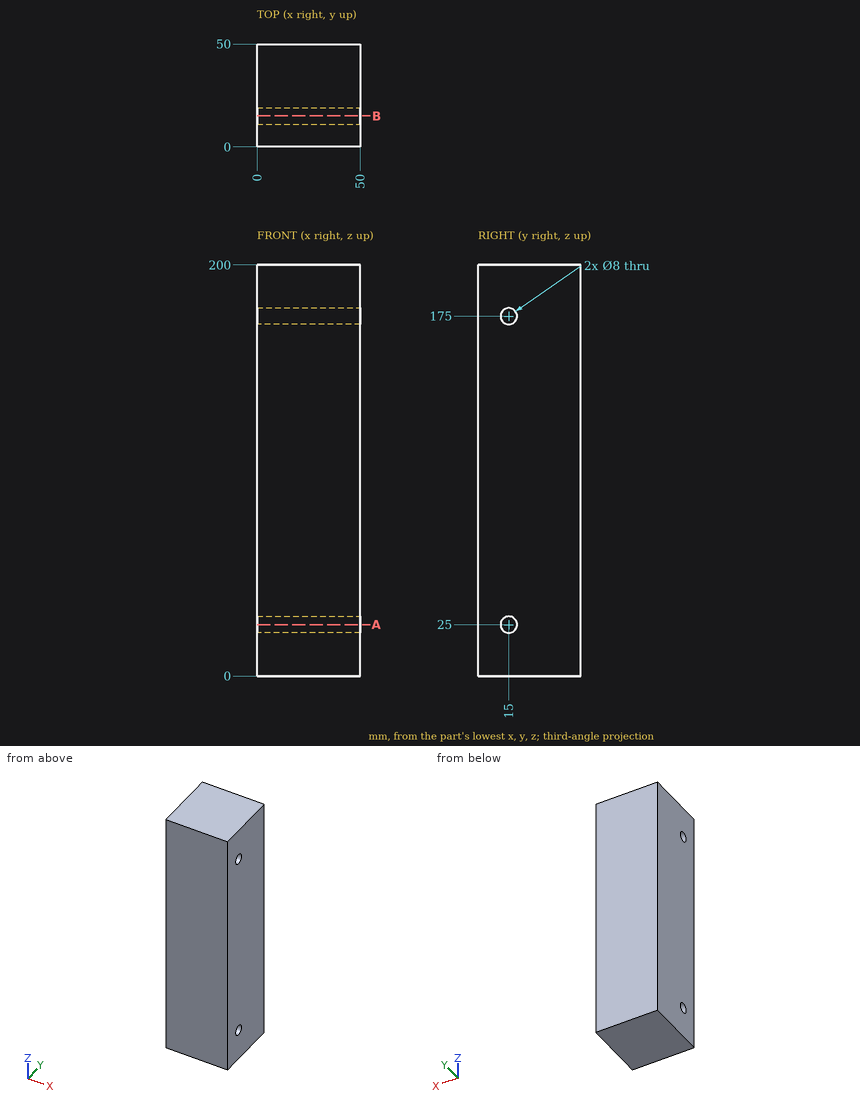
Part print with two shaded views. Sizes in mm from the minimum x, y, z corner. Coordinates: 2 decimals unless noted, no trailing zeros. Write each loop counter-clockwise with the first axis right and the second up, starting at its lowest first coordinate (ties: lowest second). Pieces come first, ordered by that corner, then holes. Notation, with made-up numbers: (-20, 60) - (4, 60) arc R20 ccw to (4, 97) - close; hole circle Ø11 at (49.5, 70). An arc over 180 degrees is marked (long way). Use a Markdown table: item, result. Add a question column.
Item 1: Drill centre lines: line 1 along Y through (x, z) = (36.5, 175); line 2 along Z through (x, y) = (16.5, 13); line 3 along Z through (x, y) = (14, 12). Where is each one in solid material? Low to high.
Item 2: Band-saw the part on B-B, the plane y = 15. Write the cut outline in (x, z).
Item 3: Drop a flat-ended pin along its axis: pin 1 (13 mm diameter, centred on y = 15, z = 25, fed in from +X). Give the stop position or say it passes through.
Item 4: Band-saw the part on A-A, the plane z = 25. Write the cut outline in (x, y), and give its area (3 significant figures).
A:
| question | item | result |
|---|---|---|
| 1 | line 1 | y = 0 to 11, 19 to 50 |
| 1 | line 2 | z = 0 to 21.54, 28.46 to 171.54, 178.46 to 200 |
| 1 | line 3 | z = 0 to 22.35, 27.65 to 172.35, 177.65 to 200 |
| 2 | outline | (0, 0) - (50, 0) - (50, 21) - (0, 21) - close; (0, 29) - (50, 29) - (50, 171) - (0, 171) - close; (0, 179) - (50, 179) - (50, 200) - (0, 200) - close |
| 3 | pin 1 | stops at x = 50 |
| 4 | outline | (0, 0) - (50, 0) - (50, 11) - (0, 11) - close; (0, 19) - (50, 19) - (50, 50) - (0, 50) - close |
| 4 | area | 2,100 mm² |
